For this review, take the finished solid that the model builds, in its own axes (mm). A direction names the side the tool comes from. Give positions to 0.01 mm unless a question says otherwise; leave off trailing zeros. Write each loop counter-clockwise with the first axis right and the second up, starting at its lowest first coordinate (ties: lowest second). Pieces come first, ordered by that corner, then holes.
Q1. For line 1 (Y direction, x = 0.9, z = 0); line 2 (Y direction, x = 3.75, z = 0); line 3 (Y direction, x = 1.25, z = 20), list the stretches that pass through material, from the lowest coordinate up.
Q2. We need section A-A (z = 0). Give the number of separate pieces and of enclosed holes in the cut face, then the cut area to 3 significant figures.
Q3. Mouldability with a two-part tool opening along Y and no side actions: class faces 1 (the cylindrical face through (0.986, -26.034, -0.521)), 2 (the cylindrical face through (-2, 0, -6)), 3 (the cylindrical face through (1, -2.4, 26.8)) as released by +Y, released by -Y, zero draft, split by the parting line, or undercut.
Q4. Machinability: for faces 4 (the flat face through (2, 16, 4)), 5 (the cylindrical face through (1, -2.4, -33.2)), which of the approach directions +Z, -Z, +X, -X, +Y, -Y give a long, thin tool a straight path to every point of the face, cutting with its end or side? Answer none if there is none.
Q5. We need section C-C (z = 30). Write out the cut boundary in (x, y).
Q6. We need section D-D (x = -1). Write out the cut boundary in (y, z).
Q7. Insertion check: P1, Ø4, axis at x = 3, y = -14.5, coming from the +Z side; P2, Ø1.5, axis at x = 1.5, y = -13, coming from the -Z side; P3, Ø5.5, axis at x = 2, y = 16.5, coming from the +Z side; P4, Ø2.5, axis at y = 30, z = 0, coming from the -X side. Each pin has a flat end and moves straight along its axis. Give the tip position at first contact, or say it passes through.
```python
from build123d import *

# Parameters (mm, degrees)
SKETCH1_R           = 35
BOSS_EXTRUDE1_DEPTH = 5
SKETCH2_R           = 1.6
CUT_EXTRUDE1_DEPTH  = 6
SKETCH3_R           = 6
BOSS_EXTRUDE2_DEPTH = 5
SKETCH6_R           = 4
CUT_EXTRUDE2_DEPTH  = 2
CUT_EXTRUDE3_DEPTH  = 2.3876


with BuildPart() as part:
    # Sketch1 → Boss-Extrude1 (new body)
    with BuildSketch(Plane(origin=(0, 0, 0), x_dir=(0, 0, -1), z_dir=(1, 0, 0))):
        Circle(SKETCH1_R)
        with BuildLine():
            Line((4, 6.92820323), (4, 24.677925359))
            ThreePointArc((4, 24.677925359), (17.67766953, 17.67766953), (24.677925359, 4))
            Line((24.677925359, 4), (6.92820323, 4))
            ThreePointArc((6.92820323, 4), (5.656854249, 5.656854249), (4, 6.92820323))
        make_face(mode=Mode.SUBTRACT)
        with BuildLine():
            Line((-4, 24.677925359), (-4, 6.92820323))
            ThreePointArc((-4, 6.92820323), (-5.656854249, 5.656854249), (-6.92820323, 4))
            Line((-6.92820323, 4), (-24.677925359, 4))
            ThreePointArc((-24.677925359, 4), (-17.67766953, 17.67766953), (-4, 24.677925359))
        make_face(mode=Mode.SUBTRACT)
        with BuildLine():
            Line((-24.677925359, -4), (-6.92820323, -4))
            ThreePointArc((-6.92820323, -4), (-5.656854249, -5.656854249), (-4, -6.92820323))
            Line((-4, -6.92820323), (-4, -24.677925359))
            ThreePointArc((-4, -24.677925359), (-17.67766953, -17.67766953), (-24.677925359, -4))
        make_face(mode=Mode.SUBTRACT)
        with BuildLine():
            Line((4, -24.677925359), (4, -6.92820323))
            ThreePointArc((4, -6.92820323), (5.656854249, -5.656854249), (6.92820323, -4))
            Line((6.92820323, -4), (24.677925359, -4))
            ThreePointArc((24.677925359, -4), (17.67766953, -17.67766953), (4, -24.677925359))
        make_face(mode=Mode.SUBTRACT)
        with BuildLine():
            Line((2.28035085, 2.1), (-2.28035085, 2.1))
            ThreePointArc((-2.28035085, 2.1), (0, -3.1), (2.28035085, 2.1))
        make_face(mode=Mode.SUBTRACT)
    extrude(amount=BOSS_EXTRUDE1_DEPTH)

    # Sketch2 → Cut-Extrude1 (cut, through all)
    with BuildSketch(Plane.ZY):
        with Locations((0, 30)):
            Circle(SKETCH2_R)
        with Locations((30, 0)):
            Circle(SKETCH2_R)
        with Locations((0, -30)):
            Circle(SKETCH2_R)
        with Locations((-30, 0)):
            Circle(SKETCH2_R)
    extrude(amount=-CUT_EXTRUDE1_DEPTH, mode=Mode.SUBTRACT)

    # Sketch3 → Boss-Extrude2 (add)
    with BuildSketch(Plane.ZY):
        Circle(SKETCH3_R)
        with BuildLine():
            Line((-2.28035085, 2.1), (2.28035085, 2.1))
            ThreePointArc((2.28035085, 2.1), (0, -3.1), (-2.28035085, 2.1))
        make_face(mode=Mode.SUBTRACT)
    extrude(amount=BOSS_EXTRUDE2_DEPTH)

    # Sketch6 → Cut-Extrude2 (cut)
    with BuildSketch(Plane.ZY):
        with Locations((0, 30)):
            Circle(SKETCH6_R)
        with Locations((30, 0)):
            Circle(SKETCH6_R)
        with Locations((0, -30)):
            Circle(SKETCH6_R)
        with Locations((-30, 0)):
            Circle(SKETCH6_R)
    extrude(amount=-CUT_EXTRUDE2_DEPTH, mode=Mode.SUBTRACT)

    # Sketch7 → Cut-Extrude3 (cut)
    with BuildSketch(Plane.ZY.offset(5)):
        with BuildLine():
            Line((-3.9116, -3.300656457), (-3.9116, 3.300656457))
            ThreePointArc((-3.9116, 3.300656457), (0, 5.1181), (3.9116, 3.300656457))
            Line((3.9116, 3.300656457), (3.9116, -3.300656457))
            ThreePointArc((3.9116, -3.300656457), (0, -5.1181), (-3.9116, -3.300656457))
        make_face()
    extrude(amount=-CUT_EXTRUDE3_DEPTH, mode=Mode.SUBTRACT)


solid = part.part
```
Computed:
1. line 1: y = -35 to -34, -26 to -3.1, 2.1 to 26, 34 to 35
1. line 2: y = -35 to -31.6, -28.4 to -3.1, 2.1 to 28.4, 31.6 to 35
1. line 3: y = -28.72 to -15, -4 to 4, 15 to 28.72
2. separate pieces: 4
2. enclosed holes: 0
2. area: 295 mm2
3. face 1: undercut
3. face 2: split by the parting line
3. face 3: undercut
4. face 4: +X, -X
4. face 5: -X
5. outline: (0, -18.03) - (5, -18.03) - (5, -1.6) - (2, -1.6) - (2, -4) - (0, -4) - close; (0, 4) - (2, 4) - (2, 1.6) - (5, 1.6) - (5, 18.03) - (0, 18.03) - close
6. outline: circle Ø12 at (0, 0); hole (2.1, -2.28) - (2.1, 2.28) arc R3.1 ccw (long way) to start
7. P1: stops at z = 32.69
7. P2: stops at z = -32.79
7. P3: stops at z = 32.19
7. P4: passes through
